Design review of the part built by this model. Coordinates are the model's own, in mm. Face numbers are marked on the shaded views. A direction names the side the tool comes from. Coordinates: 2 decimals unless noted, no trailing zeros. Loops run counter-clockwise (first coordinate to the right, second up) from the corner with the lowest first, then second, coordinate; pieces in that order, holes last. Notation, with made-up numbers: M 84,78 L 120,78 A36 cw 120,114 Z; hole C -7,-10.5 d3. An arc over 180 degrees is marked long. Write item = value, one per line. Start each with the question number.
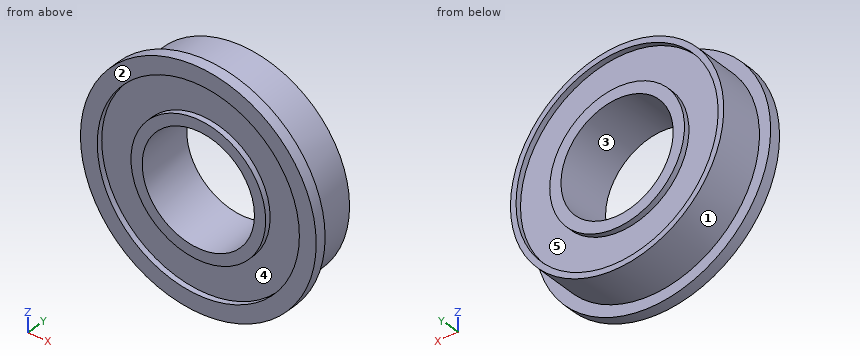
```python
from build123d import *

# Parameters (mm, degrees)
SKETCH_1_R          = 9.5
EXTRUDE_1_DEPTH     = 4
SKETCH_2_R          = 10.5
EXTRUDE_2_DEPTH     = 1
CUT_EXTRUDE_1_REACH = 7
SKETCH_3_R          = 5
SKETCH_4_R          = 9
SKETCH_4_R_2        = 6
CUT_EXTRUDE_2_DEPTH = 0.5
CUT_EXTRUDE_START   = -5
SKETCH_4_2_R        = 9
SKETCH_4_2_R_2      = 6
CUT_EXTRUDE_5_DEPTH = 0.5


with BuildPart() as part:
    # Sketch 1 → Extrude 1 (new body)
    with BuildSketch(Plane(origin=(0, 0, 0), x_dir=(1, 0, 0), z_dir=(0, 1, 0))):
        Circle(SKETCH_1_R)
    extrude(amount=EXTRUDE_1_DEPTH)

    # Sketch 2 → Extrude 2 (add)
    with BuildSketch(Plane.XZ):
        Circle(SKETCH_2_R)
    extrude(amount=EXTRUDE_2_DEPTH)

    # Sketch 3 → Cut-Extrude 1 (cut, up to next)
    with BuildSketch(Plane(origin=(0, 4, 0), x_dir=(1, 0, 0), z_dir=(0, 1, 0)), mode=Mode.PRIVATE) as cut_extrude_1_sk1:
        Circle(SKETCH_3_R)
    cut_extrude_1_tool1 = extrude(cut_extrude_1_sk1.sketch, amount=-CUT_EXTRUDE_1_REACH, mode=Mode.PRIVATE) & part.part
    add(cut_extrude_1_tool1.solids().sort_by_distance((0, 4, 0))[0], mode=Mode.SUBTRACT)

    # Sketch 4 → Cut-Extrude 2 (cut)
    with BuildSketch(Plane(origin=(0, 4, 0), x_dir=(1, 0, 0), z_dir=(0, 1, 0))):
        Circle(SKETCH_4_R)
        Circle(SKETCH_4_R_2, mode=Mode.SUBTRACT)
    extrude(amount=-CUT_EXTRUDE_2_DEPTH, mode=Mode.SUBTRACT)

    # Sketch 4_2 → Cut-Extrude 5 (cut)
    with BuildSketch(Plane(origin=(0, 4, 0), x_dir=(1, 0, 0), z_dir=(0, 1, 0)).offset(CUT_EXTRUDE_START)):
        Circle(SKETCH_4_2_R)
        Circle(SKETCH_4_2_R_2, mode=Mode.SUBTRACT)
    extrude(amount=CUT_EXTRUDE_5_DEPTH, mode=Mode.SUBTRACT)


solid = part.part
```
(1) Take a section at B-B (x = 0). State the section outline as (y, z) points, plus the area to 3 significant figures.
(2) Tool access review of the marked faces 4 and 5: name each direction out of +Z, -Z, +X, -X, +Y, -Y from which nothing blocks a thin tool from reaching the whole face with its end or side.
(3) To check wall thickness, follow L1, parallel to Z at x = 0, y = 3.9; L2, parallel to Z at x = 0, y = -0.6. State the ranges of each line that lie inside material, in increasing order.
(4) Take a section at A-A (z = 0). State the section outline as (x, y) points.
(5) Take a section at D-D (z = 7.25). State the section outline as (x, y) points.
(6) Mouldability with a two-part tool opening along Z and no side actions: class the marked faces 1, 2 and 3 as +Z half, -Z half, draft (parallel to the pull), parting line (faces both ways), or undercut.
(7) Insertion check: pin 1 (10 mm diameter, centred on x = 4, z = 8, fed in from +Y); pin 2 (3 mm diameter, centred on y = 1, z = 2.5, fed in from -X); pin 3 (3 mm diameter, centred on y = 0.5, z = -5.5, fed in from -X). Each pin has a flat end and moves straight along its axis. Give the tip position at first contact, or say it passes through.
(8) Take a section at C-C (y = 1.95). State the section outline as (x, z) points, plus the area to 3 significant figures.
Results list:
q1.outline = M -1,-10.5 L 0,-10.5 L 0,-9.5 L 4,-9.5 L 4,-9 L 3.5,-9 L 3.5,-6 L 4,-6 L 4,-5 L -1,-5 L -1,-6 L -0.5,-6 L -0.5,-9 L -1,-9 Z; M -1,5 L 4,5 L 4,6 L 3.5,6 L 3.5,9 L 4,9 L 4,9.5 L 0,9.5 L 0,10.5 L -1,10.5 L -1,9 L -0.5,9 L -0.5,6 L -1,6 Z
q1.area = 41.0 mm^2
q2.face_4 = -Y
q2.face_5 = +Y
q3.L1 = -9.5 to -9, -6 to -5, 5 to 6, 9 to 9.5
q3.L2 = -10.5 to -9, -6 to -5, 5 to 6, 9 to 10.5
q4.outline = M -10.5,-1 L -9,-1 L -9,-0.5 L -6,-0.5 L -6,-1 L -5,-1 L -5,4 L -6,4 L -6,3.5 L -9,3.5 L -9,4 L -9.5,4 L -9.5,0 L -10.5,0 Z; M 5,-1 L 6,-1 L 6,-0.5 L 9,-0.5 L 9,-1 L 10.5,-1 L 10.5,0 L 9.5,0 L 9.5,4 L 9,4 L 9,3.5 L 6,3.5 L 6,4 L 5,4 Z
q5.outline = M -7.6,-1 L -5.33,-1 L -5.33,-0.5 L 5.33,-0.5 L 5.33,-1 L 7.6,-1 L 7.6,0 L 6.14,0 L 6.14,4 L 5.33,4 L 5.33,3.5 L -5.33,3.5 L -5.33,4 L -6.14,4 L -6.14,0 L -7.6,0 Z
q6.face_1 = parting line
q6.face_2 = draft
q6.face_3 = undercut
q7.pin_1 = 4
q7.pin_2 = -10.41
q7.pin_3 = -9.67
q8.outline = C 0,0 d19; hole C 0,0 d10
q8.area = 205 mm^2
